```python
from build123d import *

# Parameters (mm, degrees)
F1_DEPTH = 4
F2_R     = 7
F3_DEPTH = 14
F4_R     = 3
F5_SIZE  = 1
F6_SIZE  = 2


with BuildPart() as f1:
    # F0 (on Top) → F1 (new body)
    with BuildSketch(Plane.XY):
        Polygon((40, 0), (0, 0), (20, -34.641016), align=None)
    extrude(amount=F1_DEPTH)

    # F2 (on face) → F3 (join)
    with BuildSketch(Plane.XY.offset(4)):
        with Locations((20, -11.547005)):
            Circle(F2_R)
    extrude(amount=F3_DEPTH)

    # F4
    f4_edges = [f1.edges().sort_by_distance(p)[0] for p in [
        (20, -34.641016, 2),
        (40, 0, 2),
        (0, 0, 2),
    ]]
    fillet(f4_edges, radius=F4_R)

    # F5
    f5_edges = [f1.edges().sort_by_distance(p)[0] for p in [
        (30, -17.320508, 4),
    ]]
    chamfer(f5_edges, length=F5_SIZE)

    # F6
    f6_edges = [f1.edges().sort_by_distance(p)[0] for p in [
        (13, -11.547005, 18),
        (13, -11.547005, 4),
    ]]
    chamfer(f6_edges, length=F6_SIZE)


solid = f1.part
```
Build history of the part. All positions in model axes, mm. A direction names the side the tool comes from. Round coordinates to 2 decimals unless told otherwise and drop trailing zeros. Order: outer loops, then holes, each group sorted by start corner. A loop starts at its lowest first (then second) coordinate and runs counter-clockwise, first axis right, second up. Notation, with made-up numbers: (-36.75, 64.5) -> (-7.75, 64.5) arc R12 ccw to (-7.75, 84.5) -> close; hole circle Ø7 at (-28, 47). An arc over 180 degrees is marked (long way). Answer in a Markdown table with one row per item.
1) Which spindle directions (+Z, -Z, +X, -X, +Y, -Y) get a long thin tool onto all of the face, cutting with end or side? Do faces 1 (the flat face through (20.2, -0.5, 3.5)), 2 (the cylindrical face through (13.007, -11.239, 10.93)). Say none if no direction does.
Values:
| item | result |
|---|---|
| face 1 | +Z, +X, -X, +Y |
| face 2 | +Z |
2) Band-saw the part on D-D on x = 6. Give the cut face in (y, z).
Values:
| item | result |
|---|---|
| outline | (-10.39, 0) -> (0, 0) -> (0, 3) -> (-1, 4) -> (-8.39, 4) -> (-10.39, 3) -> close |
3) Band-saw the part on A-A on x = 20. Give the cut face in (y, z).
Values:
| item | result |
|---|---|
| outline | (-31.64, 0) -> (0, 0) -> (0, 3) -> (-1, 4) -> (-2.55, 4) -> (-4.55, 6) -> (-4.55, 16) -> (-6.55, 18) -> (-16.55, 18) -> (-18.55, 16) -> (-18.55, 6) -> (-20.55, 4) -> (-30.64, 4) -> (-31.64, 3) -> close |
4) Band-saw the part on C-C on z = 5.5. Give the cut face in (x, y), and give its area (3 significant figures).
Values:
| item | result |
|---|---|
| outline | circle Ø15 at (20, -11.55) |
| area | 177 mm2 |
5) Wall check: L1, parallel to Z at x = 5.5, y = -2; L2, parallel to Y at x = 31.5, z = 1.5; L3, parallel to X at y = -15.5, z = 1.5. Give the ranges that are in metal, low to high.
Values:
| item | result |
|---|---|
| L1 | 0 to 4 |
| L2 | -14.72 to 0 |
| L3 | 8.95 to 31.05 |
6) Band-saw the part on B-B on y = -27.5. Give the cut face in (x, z), and give its area (3 significant figures).
Values:
| item | result |
|---|---|
| outline | (15.88, 0) -> (24.12, 0) -> (24.12, 3) -> (22.97, 4) -> (17.03, 4) -> (15.88, 3) -> close |
| area | 31.8 mm2 |
7) Pin check, flat tips, straight feed: P1, Ø1, axis at x = 10, z = 2, coming from the -Y side; P2, Ø1.5, axis at y = -13.5, z = 10, coming from the -X side; P3, Ø8, axis at y = -20.5, z = 9, coming from the -X side. Stop position of each tip, or through.
Values:
| item | result |
|---|---|
| P1 | y = -18.19 |
| P2 | x = 13.1 |
| P3 | x = 15.05 |
